from build123d import *

# Parameters (mm, degrees)
PAD_DEPTH       = 14.5
PAD001_DEPTH    = 20
PAD002_DEPTH    = 5
PAD003_DEPTH    = 5
SKETCH009_R     = 10
POCKET_DEPTH    = 135.001
SKETCH010_R     = 10
POCKET001_DEPTH = 17.001
FILLET_R        = 2.5


with BuildPart() as part:
    # Sketch → Pad (new body)
    with BuildSketch(Plane.XY):
        with BuildLine():
            Line((-25, 70), (-25, -70))
            ThreePointArc((-25, -70), (0, -95), (25, -70))
            Line((25, -25), (25, -70))
            Line((75, -25), (25, -25))
            ThreePointArc((75, -25), (100, 0), (75, 25))
            Line((75, 25), (25, 25))
            Line((25, 25), (25, 70))
            ThreePointArc((25, 70), (0, 95), (-25, 70))
        make_face()
    extrude(amount=PAD_DEPTH)

    # Sketch001 → Pad001 (join, symmetric)
    with BuildSketch(Plane.YZ):
        Polygon((-37.5, 0), (-37.5, 70), (-22.5, 70), (-22.5, 27), (22.5, 27), (22.5, 70), (37.5, 70), (37.5, 0), align=None)
    extrude(amount=PAD001_DEPTH, both=True)

    # Sketch002 → Pad002 (join, symmetric)
    with BuildSketch(Plane.YZ):
        Polygon((-37.5, 49.5), (-37.5, 14.5), (-49.5, 14.5), align=None)
        Polygon((37.5, 49.5), (37.5, 14.5), (49.5, 14.5), align=None)
    extrude(amount=PAD002_DEPTH, both=True)

    # Sketch003 → Pad003 (join, symmetric)
    with BuildSketch(Plane.XZ):
        Polygon((20, 14.5), (20, 27), (26, 27), (54, 14.5), align=None)
    extrude(amount=PAD003_DEPTH, both=True)

    # Sketch004 → Revolution (revolve)
    with BuildSketch(Plane.YZ):
        Polygon((-40, 70), (-40, 87.5), (-37.5, 90), (-22.5, 90), (-20, 87.5), (-20, 70), align=None)
    revolve(axis=Axis((0, -20, 70), (0, 1, 0)))

    # Sketch005 → Revolution001 (revolve)
    with BuildSketch(Plane.YZ):
        Polygon((20, 70), (20, 87.5), (22.5, 90), (37.5, 90), (40, 87.5), (40, 70), align=None)
    revolve(axis=Axis((0, 20, 70), (0, -1, 0)))

    # Sketch006 → Revolution002 (revolve)
    with BuildSketch(Plane.YZ):
        Polygon((-90, 14.5), (-70, 14.5), (-70, 17), (-87.5, 17), align=None)
    revolve(axis=Axis((0, -70, 14.5), (0, 0, -1)))

    # Sketch007 → Revolution003 (revolve)
    with BuildSketch(Plane.YZ):
        Polygon((50, 14.5), (70, 14.5), (70, 17), (52.5, 17), align=None)
    revolve(axis=Axis((0, 70, 14.5), (0, 0, -1)))

    # Sketch008 → Revolution004 (revolve)
    with BuildSketch(Plane.XZ):
        Polygon((55, 14.5), (75, 14.5), (75, 17), (57.5, 17), align=None)
    revolve(axis=Axis((75, 0, 14.5), (0, 0, -1)))

    # Sketch009 (on Face38 of Revolution004) → Pocket (cut, through all)
    with BuildSketch(Plane.XZ.offset(40)):
        with Locations((0, 70)):
            Circle(SKETCH009_R)
    extrude(amount=-POCKET_DEPTH, mode=Mode.SUBTRACT)

    # Sketch010 (on Face37 of Pocket) → Pocket001 (cut, through all)
    with BuildSketch(Plane.XY.offset(17)):
        with Locations((0, 70)):
            Circle(SKETCH010_R)
        with Locations((75, 0)):
            Circle(SKETCH010_R)
        with Locations((0, -70)):
            Circle(SKETCH010_R)
    extrude(amount=-POCKET001_DEPTH, mode=Mode.SUBTRACT)

    # Fillet
    fillet_edges = [part.edges().sort_by_distance(p)[0] for p in [
        (25, -25, 7.25),
        (25, 25, 7.25),
        (0, 22.5, 27),
        (0, -22.5, 27),
    ]]
    fillet(fillet_edges, radius=FILLET_R)


solid = part.part
CAD build for the part. Positions are in the model's coordinates, mm. A direction names the side the tool comes from. Coordinates: 2 decimals unless noted, no trailing zeros. Write each loop counter-clockwise with the first axis right and the second up, starting at its lowest first coordinate (ties: lowest second). Pieces come first, ordered by that corner, then holes. Notation, with made-up numbers: M 76,-35 L 104,-35 A16 cw 104,-28 Z; hole C -8,0.25 d7. An arc over 180 degrees is marked long. Return JSON: item names as keys, results as strings.
Item 1: Probe line 1 (Y direction, x = 75, z = 12.5); line 2 (Y direction, x = 10, z = 71.5); line 3 (Z direction, x = 56, y = 19.5). List the from-to ranges inside material, lowest first. Write a range as from..to.
Findings below:
{"line 1": "y = -25..-10, 10..25", "line 2": "y = -40..-20, 20..40", "line 3": "z = 0..14.5"}
Item 2: Slice it at A-A, the plane z = 39. Write the cut outline in (x, y).
Findings below:
{"outline": "M -20,-37.5 L -5,-37.5 L -5,-41.1 L 5,-41.1 L 5,-37.5 L 20,-37.5 L 20,-22.5 L -20,-22.5 Z; M -20,22.5 L 20,22.5 L 20,37.5 L 5,37.5 L 5,41.1 L -5,41.1 L -5,37.5 L -20,37.5 Z"}
Item 3: Two-plate mould, pull along Z, no slides. Class faces 1 (the flat face through (8, 78, 17)), 2 (the conical face through (-5.29, 39.88, 86.81)), 3 (the cylindrical face through (99.994, -0.55, 7.148)): +Z half, -Z half, draft (parallel to the pull), parting line (faces both ways), or undercut.
Findings below:
{"face 1": "+Z half", "face 2": "undercut", "face 3": "draft"}
Item 4: Slice it at B-B, the plane y = 0. Write the cut outline in (x, z).
Findings below:
{"outline": "M -25,0 L 65,0 L 65,17 L 57.5,17 L 55,14.5 L 54,14.5 L 26,27 L -20,27 L -20,14.5 L -25,14.5 Z; M 85,0 L 100,0 L 100,14.5 L 95,14.5 L 92.5,17 L 85,17 Z"}
Item 5: Which spindle directions (+Z, -Z, +X, -X, +Y, -Y) get a long thin tool onto all of the face, cutting with end or side? Do faces 4 (the flat face through (8, -62, 17)), 5 (the conical face through (-5.304, 53.159, 16.844)), 6 (the flat face through (-20, 1, 24)), 7 (the flat face through (33, 5, 19)), 8 (the flat face through (33, -5, 19)). Say none if no direction does.
Findings below:
{"face 4": "+Z, +X, -X, -Y", "face 5": "+Z", "face 6": "+Z, -X, +Y, -Y", "face 7": "+Z, +Y", "face 8": "+Z, -Y"}
Item 6: Drop flat-ended pins along their axis: pin 1 Ø4.5 at (y, z) = (-49.5, 7) entering from +X; pin 2 Ø10 at (x, z) = (39, 21) entering from -Y; pin 3 Ø17.5 at (x, z) = (6, 68) entering from -Y. Give the stop position or say it passes through.
Findings below:
{"pin 1": "stops at x = 25", "pin 2": "stops at y = -5", "pin 3": "stops at y = -40"}
Item 7: Slice it at D-D, the plane x = 47. Write the cut outline in (y, z) (3 decimals).
Findings below:
{"outline": "M -25,0 L 25,0 L 25,14.5 L 5,14.5 L 5,17.625 L -5,17.625 L -5,14.5 L -25,14.5 Z"}
Item 8: Slice it at C-C, the plane x = 0. State how many separate pieces and enclosed holes the cut face has, and give its area (3 significant figures).
Findings below:
{"separate pieces": "5", "enclosed holes": "0", "area": "5,090 mm2"}
